Geometry check sheet. Reference: the model listing, model coordinates, mm. A direction names the side the tool comes from. Round coordinates to 2 decimals unless told otherwise and drop trailing zeros. Loops run counter-clockwise (first coordinate to the right, second up) from the corner with the lowest first, then second, coordinate; pieces in that order, holes last. Notation, with made-up numbers: (54.5, 73) - (61.5, 73) arc R20 ccw to (61.5, 85) - close; hole circle Ø8 at (80.25, 65.5). An arc over 180 degrees is marked (long way). Answer in a Markdown table with one row per item. Add a question column.
```python
from build123d import *

# Parameters (mm, degrees)
SKETCH1_R           = 79.502
SKETCH1_R_2         = 39.751
BOSS_EXTRUDE1_DEPTH = 4.7625


with BuildPart() as part:
    # Sketch1 → Boss-Extrude1 (new body)
    with BuildSketch(Plane.XY):
        Circle(SKETCH1_R)
        with BuildLine():
            Line((-72.875871206, -6.35), (-45.661577951, -6.35))
            ThreePointArc((-45.661577951, -6.35), (-32.598329719, -32.598329719), (-6.35, -45.661577951))
            Line((-6.35, -45.661577951), (-6.35, -72.875871206))
            ThreePointArc((-6.35, -72.875871206), (-51.726275257, -51.726275257), (-72.875871206, -6.35))
        make_face(mode=Mode.SUBTRACT)
        with BuildLine():
            Line((45.661577951, -6.35), (72.875871206, -6.35))
            ThreePointArc((72.875871206, -6.35), (51.726275257, -51.726275257), (6.35, -72.875871206))
            Line((6.35, -72.875871206), (6.35, -45.661577951))
            ThreePointArc((6.35, -45.661577951), (32.598329719, -32.598329719), (45.661577951, -6.35))
        make_face(mode=Mode.SUBTRACT)
        with BuildLine():
            Line((-6.35, 72.875871206), (-6.35, 45.661577951))
            ThreePointArc((-6.35, 45.661577951), (-32.598329719, 32.598329719), (-45.661577951, 6.35))
            Line((-45.661577951, 6.35), (-72.875871206, 6.35))
            ThreePointArc((-72.875871206, 6.35), (-51.726275257, 51.726275257), (-6.35, 72.875871206))
        make_face(mode=Mode.SUBTRACT)
        Circle(SKETCH1_R_2, mode=Mode.SUBTRACT)
        with BuildLine():
            ThreePointArc((45.661577951, 6.35), (32.598329719, 32.598329719), (6.35, 45.661577951))
            Line((6.35, 45.661577951), (6.35, 72.875871206))
            ThreePointArc((6.35, 72.875871206), (51.726275257, 51.726275257), (72.875871206, 6.35))
            Line((72.875871206, 6.35), (45.661577951, 6.35))
        make_face(mode=Mode.SUBTRACT)
    extrude(amount=BOSS_EXTRUDE1_DEPTH)


solid = part.part
```
Q1. Cross-section at C-C, the plane z = 3.1. Enter the section's corners in (x, y), plus the area to 3 significant figures.
Q2. Set-up check for faces 4 (the flat face through (-18, 36, 0)), 5 (the flat face through (59, 6.35, 2)): record each of +Z, -Z, +X, -X, +Y, -Y from which the full face is reachable in a straight line by a thin tool's end or side.
Q3. Scan lines: line 1 (Y direction, x = 50, z = 0.8); line 2 (Y direction, x = 51, z = 1.1); line 3 (X direction, y = 16, z = 3.35). Record each from-to range of solid material in increasing order. Write a range as from..to.
Q4. Release check for a two-part mould opening along Y. For faces 1 (the cylindrical face through (51.22, 52.23, 2.35)), 2 (the cylindrical face through (-17.234, -77.611, 2.348)), 3 (the flat face through (-18, 36, 4.762)) record: +Y half, -Y half, draft (parallel to the pull), parting line (faces both ways), or undercut.
Q5. Cross-section at D-D, the plane x = 37.5. Enter the section's corners in (y, z).
Q6. Depth check by flat-ended pin: P1, Ø1, axis at y = -43, z = 0.5, coming from the +X side; P2, Ø1.4, axis at x = 64.5, z = 3.5, coming from the +Y side; P3, Ø1.4, axis at x = -59.5, z = 3.5, coming from the +Y side. Enter the tip coordinate at first touch or a pass-through.
Q7. Cross-section at A-A, the plane x = 0. Enter the section's corners in (y, z), plus the area to 3 significant figures.
Check sheet entries:
| question | item | result |
|---|---|---|
| 1 | outline | circle Ø159 at (0, 0); hole (-72.88, -6.35) arc R73.15 ccw to (-6.35, -72.88) - (-6.35, -45.66) arc R46.1 cw to (-45.66, -6.35) - close; hole (-72.88, 6.35) - (-45.66, 6.35) arc R46.1 cw to (-6.35, 45.66) - (-6.35, 72.88) arc R73.15 ccw to start; hole circle Ø79.5 at (0, 0); hole (6.35, -72.88) arc R73.15 ccw to (72.88, -6.35) - (45.66, -6.35) arc R46.1 cw to (6.35, -45.66) - close; hole (6.35, 45.66) arc R46.1 cw to (45.66, 6.35) - (72.88, 6.35) arc R73.15 ccw to (6.35, 72.88) - close |
| 1 | area | 6,130 mm² |
| 2 | face 4 | -Z, +X, -X, +Y, -Y |
| 2 | face 5 | +Z, -Z |
| 3 | line 1 | -61.81..-53.4, -6.35..6.35, 53.4..61.81 |
| 3 | line 2 | -60.99..-52.44, -6.35..6.35, 52.44..60.99 |
| 3 | line 3 | -77.88..-71.38, -43.24..-36.39, 36.39..43.24, 71.38..77.88 |
| 4 | face 1 | undercut |
| 4 | face 2 | parting line |
| 4 | face 3 | draft |
| 5 | outline | (-70.1, 0) - (-62.81, 0) - (-62.81, 4.76) - (-70.1, 4.76) - close; (-26.82, 0) - (-13.19, 0) - (-13.19, 4.76) - (-26.82, 4.76) - close; (13.19, 0) - (26.82, 0) - (26.82, 4.76) - (13.19, 4.76) - close; (62.81, 0) - (70.1, 0) - (70.1, 4.76) - (62.81, 4.76) - close |
| 6 | P1 | x = 67.19 |
| 6 | P2 | y = 47.44 |
| 6 | P3 | y = 53.51 |
| 7 | outline | (-79.5, 0) - (-39.75, 0) - (-39.75, 4.76) - (-79.5, 4.76) - close; (39.75, 0) - (79.5, 0) - (79.5, 4.76) - (39.75, 4.76) - close |
| 7 | area | 379 mm² |
